Source: CAD feature listing. Evaluate the final solid. Frame: model axes, mm. Face numbers are marked on the shaded views. Give positions to 0.01 mm unless a question says otherwise; leave off trailing zeros. Order: outer loops, then holes, each group sorted by start corner. A loop starts at its lowest first (then second) coordinate and runs counter-clockwise, first axis right, second up.
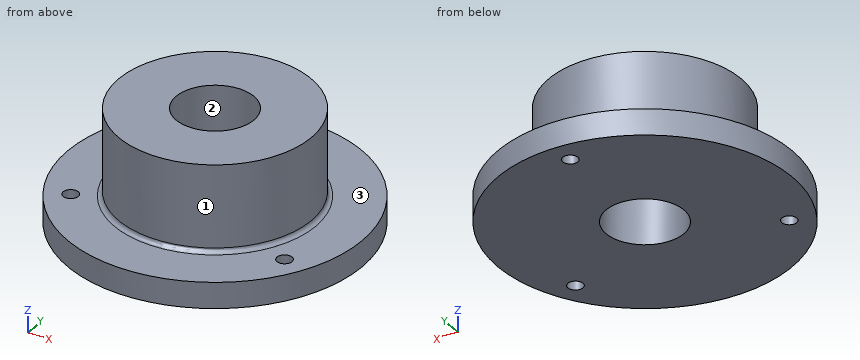
```python
from build123d import *

# Parameters (mm, degrees)
SKETCH_1_R                 = 34
EXTRUDE_252_DEPTH          = 6
SKETCH_2_R                 = 22.25
EXTRUDE_346_DEPTH          = 20
SKETCH_4_R                 = 1.75
CUT_EXTRUDE_656_DEPTH      = 53.076866265
FILLET_1_R                 = 1
CUT_EXTRUDE_770_DEPTH      = 55.662601475
CUT_EXTRUDE_770_DEPTH_BACK = 55.662601475
SKETCH_3_R                 = 9


with BuildPart() as part:
    # 草图1 → Extrude 252 (new body)
    with BuildSketch(Plane.XY):
        Circle(SKETCH_1_R)
    extrude(amount=EXTRUDE_252_DEPTH)

    # 草图2 → Extrude 346 (add)
    with BuildSketch(Plane.XY.offset(6)):
        Circle(SKETCH_2_R)
    extrude(amount=EXTRUDE_346_DEPTH)

    # 草图4 → Cut-Extrude 656 (cut, through all)
    with BuildSketch(Plane.XY.offset(6)):
        with Locations((0, 28.5)):
            Circle(SKETCH_4_R)
        with Locations((24.681724008, -14.25)):
            Circle(SKETCH_4_R)
        with Locations((-24.681724008, -14.25)):
            Circle(SKETCH_4_R)
    extrude(amount=-CUT_EXTRUDE_656_DEPTH, mode=Mode.SUBTRACT)

    # 圆角1
    fillet_1_edges = [part.edges().sort_by_distance(p)[0] for p in [
        (-22.25, 0, 6),
    ]]
    fillet(fillet_1_edges, radius=FILLET_1_R)

    # 草图3 → Cut-Extrude 770 (cut, two sides: drawn at the far end of the back side and taken through both)
    with BuildSketch(Plane.XY.offset(26).offset(-CUT_EXTRUDE_770_DEPTH_BACK)):
        Circle(SKETCH_3_R)
    extrude(amount=CUT_EXTRUDE_770_DEPTH + CUT_EXTRUDE_770_DEPTH_BACK, mode=Mode.SUBTRACT)


solid = part.part
```
1) Pin query (flat end, axial travel): pin 1 (6 mm diameter, centred on x = -25, y = -14, fed in from +Z); pin 2 (2 mm diameter, centred on x = 0, y = 28.5, fed in from +Z); pin 3 (1.5 mm diameter, centred on x = -12, z = 20.5, fed in from -Y); pin 4 (2 mm diameter, centred on x = 8.5, z = 17.5, fed in from +Y). Return the tip coordinate at first contact, or that it passes through.
Report:
pin 1: stops at z = 6
pin 2: passes through
pin 3: stops at y = -19.2
pin 4: stops at y = 20.95
2) Section query B-B, the plane x = 0. Return the cut outline in (y, z), and give its area (3 significant figures).
Report:
outline: (-34, 0) - (-9, 0) - (-9, 26) - (-22.25, 26) - (-22.25, 7) arc R1 cw to (-23.25, 6) - (-34, 6) - close; (9, 0) - (26.75, 0) - (26.75, 6) - (23.25, 6) arc R1 cw to (22.25, 7) - (22.25, 26) - (9, 26) - close; (30.25, 0) - (34, 0) - (34, 6) - (30.25, 6) - close
area: 809 mm2
3) Material intervals for L1, parallel to Y at x = 0, z = 2.15; L2, parallel to Y at x = 0, z = 11.75; L3, parallel to Z at x = -6.5, y = -31, sorted ascending.
Report:
L1: y = -34 to -9, 9 to 26.75, 30.25 to 34
L2: y = -22.25 to -9, 9 to 22.25
L3: z = 0 to 6
4) Draft query along Y for the marked faces 1, 2 and 3. Return one class per face: +Y half, -Y half, draft (parallel to the pull), parting line (faces both ways), or undercut.
Report:
face 1: parting line
face 2: undercut
face 3: draft
5) Section query D-D, the plane z = 15.75. Return the cut outline in (x, y), and give its area (3 significant figures).
Report:
outline: circle Ø44.5 at (0, 0); hole circle Ø18 at (0, 0)
area: 1,300 mm2
6) Section query A-A, the plane y = 0. Return the cut outline in (x, z).
Report:
outline: (-34, 0) - (-9, 0) - (-9, 26) - (-22.25, 26) - (-22.25, 7) arc R1 cw to (-23.25, 6) - (-34, 6) - close; (9, 0) - (34, 0) - (34, 6) - (23.25, 6) arc R1 cw to (22.25, 7) - (22.25, 26) - (9, 26) - close
7) Section query C-C, the plane x = -24.5. Return the cut outline in (y, z), and give its area (3 significant figures).
Report:
outline: (-23.57, 0) - (-15.99, 0) - (-15.99, 6) - (-23.57, 6) - close; (-12.51, 0) - (23.57, 0) - (23.57, 6) - (-12.51, 6) - close
area: 262 mm2
